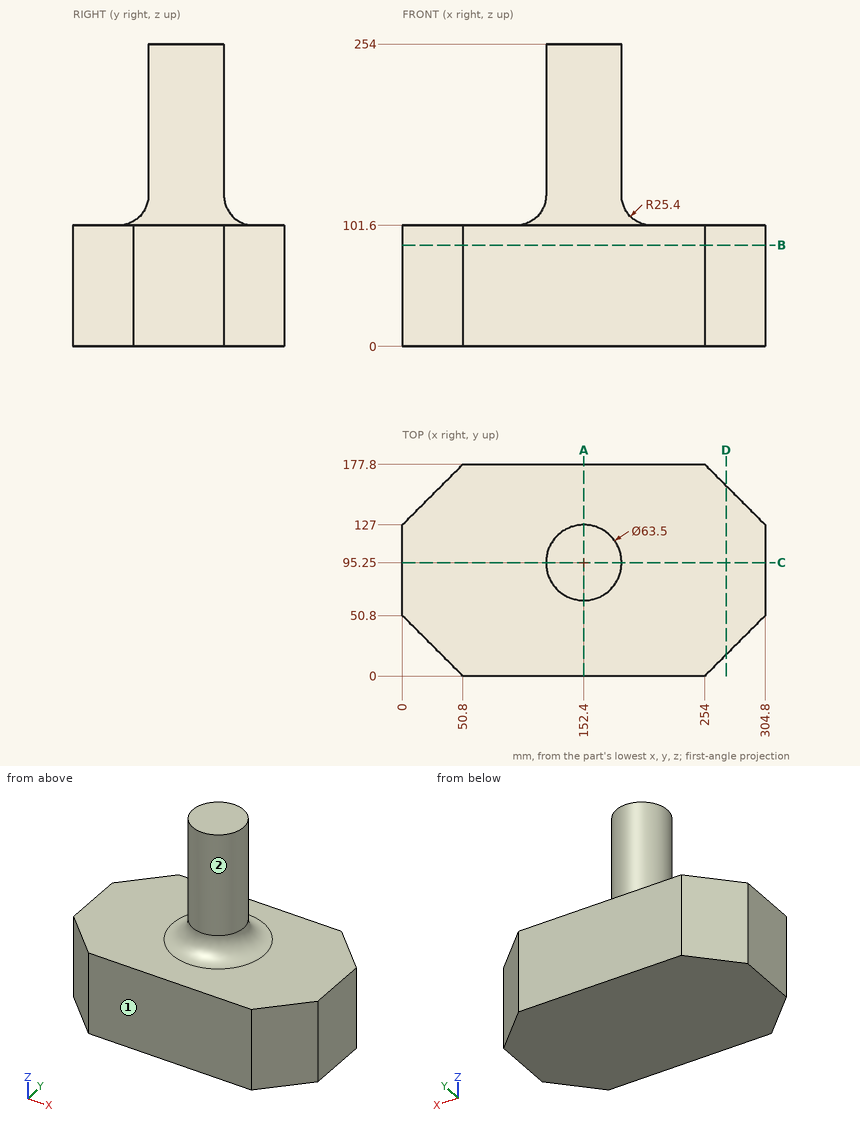
Source: three-view drawing plus pictorial views. Frame: mm from the lowest corner of the part. A direction names the side the tool comes from. Round coordinates to 2 decimals unless told otherwise and drop trailing zeros. Loops run counter-clockwise (first coordinate to the right, second up) from the corner with the lowest first, then second, coordinate; pieces in that order, holes last.
Q1. Section A-A, the plane x = 152.4. Return loops of the section in (y, z), plus the area to 3 significant figures.
Q2. Access query for the marked faces 1 and 2. Directions: +Z, -Z, +X, -X, +Y, -Y. A direction counts if a zero-diameter tool reaches every point of the face in a straight line with its end or side. Return the directions, or none.
Q3. First-contact query: P1, Ø4, axis at x = 272.5, z = 46.5, coming from the +Y side; P2, Ø8, axis at y = 94, z = 171, coming from the +X side. Flat tips, straight axial feed; report the tip coordinate or a pass-through.
Q4. Section C-C, the plane y = 95.25. Return loops of the section in (x, z), plus the area to 3 significant figures.
Q5. Ray query, line 1 (Z direction, x = 186.5, y = 162.5); line 2 (Y direction, x = 28.5, z = 88); line 3 (Y direction, x = 149, z = 202). Return the intervals inside material, ascending.
Q6. Section D-D, the plane x = 272. Return loops of the section in (y, z).
Q7. Section B-B, the plane z = 85. Return loops of the section in (x, y).
Solutions:
1. outline: (0, 0) - (177.8, 0) - (177.8, 101.6) - (152.4, 101.6) arc R25.4 cw to (127, 127) - (127, 254) - (63.5, 254) - (63.5, 127) arc R25.4 cw to (38.1, 101.6) - (0, 101.6) - close
1. area: 28,000 mm2
2. face 1: +Z, -Z, +X, -X, -Y
2. face 2: +Z
3. P1: stops at y = 161.3
3. P2: stops at x = 184.15
4. outline: (0, 0) - (304.8, 0) - (304.8, 101.6) - (209.55, 101.6) arc R25.4 cw to (184.15, 127) - (184.15, 254) - (120.65, 254) - (120.65, 127) arc R25.4 cw to (95.25, 101.6) - (0, 101.6) - close
4. area: 40,900 mm2
5. line 1: z = 0 to 101.6
5. line 2: y = 22.3 to 155.5
5. line 3: y = 63.68 to 126.82
6. outline: (18, 0) - (159.8, 0) - (159.8, 101.6) - (18, 101.6) - close
7. outline: (0, 50.8) - (50.8, 0) - (254, 0) - (304.8, 50.8) - (304.8, 127) - (254, 177.8) - (50.8, 177.8) - (0, 127) - close
